from build123d import *

# Parameters (mm, degrees)
SKETCH1_W           = 19.05
SKETCH1_H           = 19.05
BOSS_EXTRUDE1_DEPTH = 711.2
CUT_EXTRUDE1_REACH  = 713.2
SKETCH2_W           = 12.7
SKETCH2_H           = 12.7


with BuildPart() as part:
    # Sketch1 → Boss-Extrude1 (new body)
    with BuildSketch(Plane.XY):
        Rectangle(SKETCH1_W, SKETCH1_H)
    extrude(amount=-BOSS_EXTRUDE1_DEPTH)

    # Sketch2 → Cut-Extrude1 (cut, up to next)
    with BuildSketch(Plane.XY, mode=Mode.PRIVATE) as cut_extrude1_sk1:
        Rectangle(SKETCH2_W, SKETCH2_H)
    cut_extrude1_tool1 = extrude(cut_extrude1_sk1.sketch, amount=-CUT_EXTRUDE1_REACH, mode=Mode.PRIVATE) & part.part
    add(cut_extrude1_tool1.solids().sort_by_distance((0, 0, 0))[0], mode=Mode.SUBTRACT)


solid = part.part
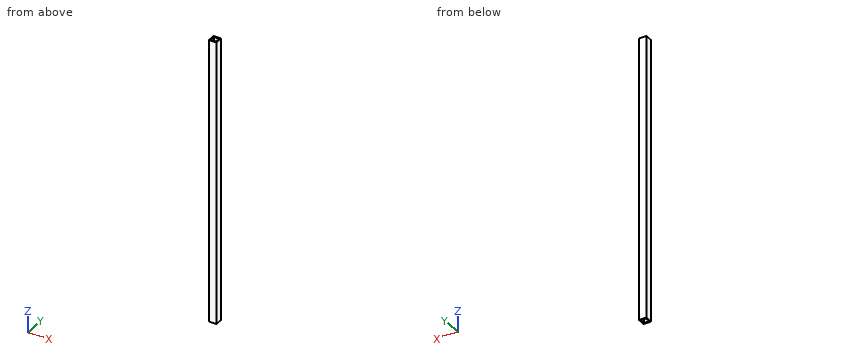
Could you check a few things on this model? Use its own coordinates, in mm. Round coordinates to 2 decimals unless told otherwise and drop trailing zeros. Order: outer loops, then holes, each group sorted by start corner. A loop starts at its lowest first (then second) coordinate and runs counter-clockwise, first axis right, second up.
(1) Imagine slicing it at A-A (x = 3). Write out the boundary of the cut face in (y, z) (3 decimals).
Response values:
outline: (-9.525, -711.2) - (-6.35, -711.2) - (-6.35, 0) - (-9.525, 0) - close; (6.35, -711.2) - (9.525, -711.2) - (9.525, 0) - (6.35, 0) - close
(2) Imagine slicing it at C-C (z = -394.5). Write out the boundary of the cut face in (x, y) (3 decimals).
Response values:
outline: (-9.525, -9.525) - (9.525, -9.525) - (9.525, 9.525) - (-9.525, 9.525) - close; hole (-6.35, -6.35) - (6.35, -6.35) - (6.35, 6.35) - (-6.35, 6.35) - close
(3) Please list where this line runs through material, in increasing order: line 1 along X through (y, z) = (-2.5, -225.5) (3 decimals).
Response values:
line 1: x = -9.525 to -6.35, 6.35 to 9.525
(4) I'm going to push a flat-ended pin straight in: pin 1 (5 mm diameter, centred on x = 1.5, y = -4.5, fed in from +Z). Where does the tip first touch, or does it pass through?
Response values:
pin 1: stops at z = 0
